The model under review builds one solid part; all positions refer to its coordinate system, in mm. A direction names the side the tool comes from. Give positions to 0.01 mm unless a question says otherwise; leave off trailing zeros. Write each question's results on one line, items separated by ' | '. Start each with the question number.
from build123d import *

# Parameters (mm, degrees)
SKETCH1_R           = 39
SKETCH1_R_2         = 1.5635
SKETCH1_R_3         = 7.5
BOSS_EXTRUDE1_DEPTH = 1
BOSS_EXTRUDE2_START = 9
SKETCH1_3_R         = 27.69
SKETCH1_3_R_2       = 1.5635
SKETCH1_3_R_3       = 7.5
BOSS_EXTRUDE2_DEPTH = 9
SKETCH2_R           = 3
SKETCH2_R_2         = 1.5635
CUT_EXTRUDE1_DEPTH  = 3
SKETCH1_4_R         = 7.5
SKETCH1_4_R_2       = 7
BOSS_EXTRUDE3_DEPTH = 1
BOSS_EXTRUDE4_START = 5
SKETCH1_5_R         = 7.5
SKETCH1_5_R_2       = 7
BOSS_EXTRUDE4_DEPTH = 5
SKETCH3_R           = 1.925
CUT_EXTRUDE2_DEPTH  = 4


with BuildPart() as part:
    # Sketch1 → Boss-Extrude1 (new body)
    with BuildSketch(Plane(origin=(0, 0, 0), x_dir=(1, 0, 0), z_dir=(0, 1, 0))):
        with Locations(Location((0, 0, 0), (0, 0, 270))):
            Circle(SKETCH1_R)
        with Locations(Location((22.5, 0, 0), (0, 0, 270))):
            Circle(SKETCH1_R_2, mode=Mode.SUBTRACT)
        with Locations(Location((15.909902577, -15.909902577, 0), (0, 0, 270))):
            Circle(SKETCH1_R_2, mode=Mode.SUBTRACT)
        with Locations(Location((0, -22.5, 0), (0, 0, 270))):
            Circle(SKETCH1_R_2, mode=Mode.SUBTRACT)
        with Locations(Location((-15.909902577, -15.909902577, 0), (0, 0, 270))):
            Circle(SKETCH1_R_2, mode=Mode.SUBTRACT)
        with Locations(Location((-22.5, 0, 0), (0, 0, 270))):
            Circle(SKETCH1_R_2, mode=Mode.SUBTRACT)
        with Locations(Location((-15.909902577, 15.909902577, 0), (0, 0, 270))):
            Circle(SKETCH1_R_2, mode=Mode.SUBTRACT)
        with Locations(Location((0, 22.5, 0), (0, 0, 270))):
            Circle(SKETCH1_R_2, mode=Mode.SUBTRACT)
        with Locations(Location((15.909902577, 15.909902577, 0), (0, 0, 270))):
            Circle(SKETCH1_R_2, mode=Mode.SUBTRACT)
        with Locations(Location((0, 0, 0), (0, 0, 270))):
            Circle(SKETCH1_R_3, mode=Mode.SUBTRACT)
    extrude(amount=-BOSS_EXTRUDE1_DEPTH)

    # Sketch1_3 → Boss-Extrude2 (add)
    with BuildSketch(Plane(origin=(0, 0, 0), x_dir=(1, 0, 0), z_dir=(0, 1, 0)).offset(BOSS_EXTRUDE2_START)):
        with Locations(Location((0, 0, 0), (0, 0, 270))):
            Circle(SKETCH1_3_R)
        with Locations(Location((22.5, 0, 0), (0, 0, 270))):
            Circle(SKETCH1_3_R_2, mode=Mode.SUBTRACT)
        with Locations(Location((15.909902577, -15.909902577, 0), (0, 0, 270))):
            Circle(SKETCH1_3_R_2, mode=Mode.SUBTRACT)
        with Locations(Location((0, -22.5, 0), (0, 0, 270))):
            Circle(SKETCH1_3_R_2, mode=Mode.SUBTRACT)
        with Locations(Location((-15.909902577, -15.909902577, 0), (0, 0, 270))):
            Circle(SKETCH1_3_R_2, mode=Mode.SUBTRACT)
        with Locations(Location((-22.5, 0, 0), (0, 0, 270))):
            Circle(SKETCH1_3_R_2, mode=Mode.SUBTRACT)
        with Locations(Location((-15.909902577, 15.909902577, 0), (0, 0, 270))):
            Circle(SKETCH1_3_R_2, mode=Mode.SUBTRACT)
        with Locations(Location((0, 22.5, 0), (0, 0, 270))):
            Circle(SKETCH1_3_R_2, mode=Mode.SUBTRACT)
        with Locations(Location((15.909902577, 15.909902577, 0), (0, 0, 270))):
            Circle(SKETCH1_3_R_2, mode=Mode.SUBTRACT)
        with Locations(Location((0, 0, 0), (0, 0, 270))):
            Circle(SKETCH1_3_R_3, mode=Mode.SUBTRACT)
    extrude(amount=-BOSS_EXTRUDE2_DEPTH)

    # Sketch2 → Cut-Extrude1 (cut)
    # profile 1 of 4: a face of its own
    with BuildSketch(Plane(origin=(0, 9, 0), x_dir=(1, 0, 0), z_dir=(0, 1, 0))):
        with Locations(Location((-15.909902577, 15.909902577, 0), (0, 0, 270))):
            Circle(SKETCH2_R)
        with Locations(Location((-15.909902577, 15.909902577, 0), (0, 0, 270))):
            Circle(SKETCH2_R_2, mode=Mode.SUBTRACT)
    # profile 2 of 4: a face of its own
    with BuildSketch(Plane(origin=(0, 9, 0), x_dir=(1, 0, 0), z_dir=(0, 1, 0))):
        with Locations(Location((15.909902577, 15.909902577, 0), (0, 0, 270))):
            Circle(SKETCH2_R)
        with Locations(Location((15.909902577, 15.909902577, 0), (0, 0, 270))):
            Circle(SKETCH2_R_2, mode=Mode.SUBTRACT)
    # profile 3 of 4: a face of its own
    with BuildSketch(Plane(origin=(0, 9, 0), x_dir=(1, 0, 0), z_dir=(0, 1, 0))):
        with Locations(Location((-15.909902577, -15.909902577, 0), (0, 0, 270))):
            Circle(SKETCH2_R)
        with Locations(Location((-15.909902577, -15.909902577, 0), (0, 0, 270))):
            Circle(SKETCH2_R_2, mode=Mode.SUBTRACT)
    # profile 4 of 4: a face of its own
    with BuildSketch(Plane(origin=(0, 9, 0), x_dir=(1, 0, 0), z_dir=(0, 1, 0))):
        with Locations(Location((15.909902577, -15.909902577, 0), (0, 0, 270))):
            Circle(SKETCH2_R)
    extrude(amount=-CUT_EXTRUDE1_DEPTH, mode=Mode.SUBTRACT)

    # Sketch1_4 → Boss-Extrude3 (add)
    with BuildSketch(Plane(origin=(0, 0, 0), x_dir=(1, 0, 0), z_dir=(0, 1, 0))):
        with Locations(Location((0, 0, 0), (0, 0, 270))):
            Circle(SKETCH1_4_R)
        with Locations(Location((0, 0, 0), (0, 0, 270))):
            Circle(SKETCH1_4_R_2, mode=Mode.SUBTRACT)
    extrude(amount=-BOSS_EXTRUDE3_DEPTH)

    # Sketch1_5 → Boss-Extrude4 (add)
    with BuildSketch(Plane(origin=(0, 0, 0), x_dir=(1, 0, 0), z_dir=(0, 1, 0)).offset(BOSS_EXTRUDE4_START)):
        with Locations(Location((0, 0, 0), (0, 0, 270))):
            Circle(SKETCH1_5_R)
        with Locations(Location((0, 0, 0), (0, 0, 270))):
            Circle(SKETCH1_5_R_2, mode=Mode.SUBTRACT)
    extrude(amount=-BOSS_EXTRUDE4_DEPTH)

    # Sketch3 → Cut-Extrude2 (cut)
    with BuildSketch(Plane.XZ.offset(1)):
        with Locations(Location((22.5, 0, 0), (0, 0, 270))):
            Circle(SKETCH3_R)
        with Locations(Location((0, -22.5, 0), (0, 0, 270))):
            Circle(SKETCH3_R)
        with Locations(Location((-22.5, 0, 0), (0, 0, 270))):
            Circle(SKETCH3_R)
        with Locations(Location((0, 22.5, 0), (0, 0, 270))):
            Circle(SKETCH3_R)
    extrude(amount=-CUT_EXTRUDE2_DEPTH, mode=Mode.SUBTRACT)


solid = part.part
(1) Machinability: for faces 1 (the cylindrical face through (-24.38, 0.97, 0.42)), 2 (the flat face through (27, 0, 8)), 3 (the flat face through (-6, 9, 6)), which of the approach directions +Z, -Z, +X, -X, +Y, -Y give a long, thin tool a straight path to every point of the face, cutting with its end or side? Answer none if there is none.
(2) Clearance check with flat-ended pins moving along their axes: P1, Ø3, axis at x = 15.91, z = -15.91, coming from the +Y side; P2, Ø1, axis at x = 21.5, z = -26.5, coming from the +Y side; P3, Ø3.5, axis at x = -15.91, z = 15.91, coming from the +Y side; P4, Ø2, axis at x = -11, y = 6.5, coming from the +Z side. State where each tip first meets the part, or that it passes through.
(3) Add section A-A (z = 0). Give the number of separate pieces and of enclosed holes in the cut face, then the cut area to 3 significant figures.
(4) Draft analysis for pull direction Z (two halves, no side actions). For faces 4 (the flat face through (-8, -1, -1)), 5 (the cylindrical face through (38.668, -0.493, -5.077)), 6 (the cylindrical face through (-18.84, 7.52, 15.26)), state which applies: pulls with the +Z half, pulls with the -Z half, needs draft (parallel to the pull), parting line crosses it, or undercut.
(5) Wall thickness on L1, parallel to Z at x = -17, y = 4.25; L2, parallel to Z at x = -1, y = 4.25; L3, parallel to X at y = 3.5, z = 16: over which ranges is each line inside the solid? List them lowest first.
Calculated:
1) face 1: -Y | face 2: +Y | face 3: +Z, -Z, +X, -X, +Y
2) P1: passes through | P2: stops at y = 0 | P3: stops at y = 6 | P4: stops at z = 25.82
3) separate pieces: 4 | enclosed holes: 0 | area: 364 mm²
4) face 4: needs draft | face 5: parting line crosses it | face 6: undercut
5) L1: z = -21.86 to -17.03, -14.79 to 14.79, 17.03 to 21.86 | L2: z = -27.67 to -23.7, -21.3 to -6.93, 6.93 to 21.3, 23.7 to 27.67 | L3: x = -22.6 to -17.47, -14.35 to 14.35, 17.47 to 22.6
